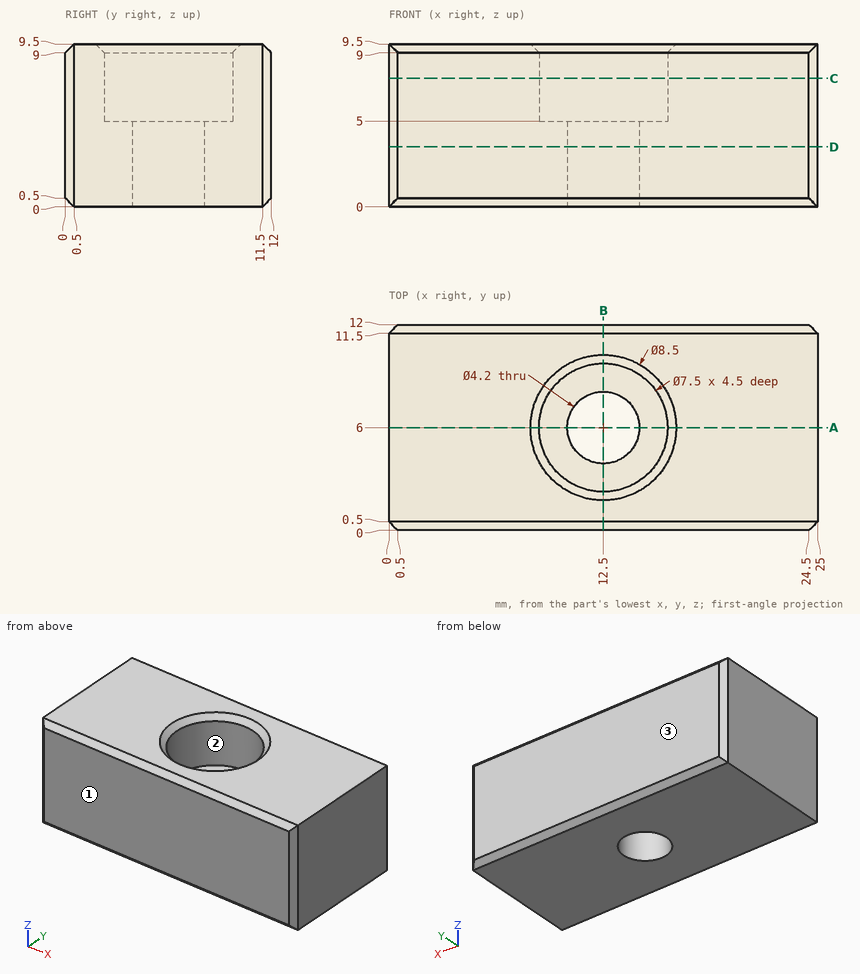
Here's the drawing with two shaded views (mm, measured from the low corner). I have some questions. Round coordinates to 2 decimals unless told otherwise and drop trailing zeros. Write each loop counter-clockwise with the first axis right and the second up, starting at its lowest first coordinate (ties: lowest second). Pieces come first, ordered by that corner, then holes.
(1) Suppose I cut it at C-C on z = 7.5. Write out the boundary of the cut face in (x, y).
Findings below:
outline: (0, 0.5) - (0.5, 0) - (24.5, 0) - (25, 0.5) - (25, 11.5) - (24.5, 12) - (0.5, 12) - (0, 11.5) - close; hole circle Ø7.5 at (12.5, 6)
(2) Suppose I cut it at D-D on z = 3.5. Write out the boundary of the cut face in (x, y), and give its area (3 significant figures).
Findings below:
outline: (0, 0.5) - (0.5, 0) - (24.5, 0) - (25, 0.5) - (25, 11.5) - (24.5, 12) - (0.5, 12) - (0, 11.5) - close; hole circle Ø4.2 at (12.5, 6)
area: 286 mm2
(3) Suppose I cut it at B-B on x = 12.5. Write out the boundary of the cut face in (y, z), and give its area (3 significant figures).
Findings below:
outline: (0, 0.5) - (0.5, 0) - (3.9, 0) - (3.9, 5) - (2.25, 5) - (2.25, 9) - (1.75, 9.5) - (0.5, 9.5) - (0, 9) - close; (8.1, 0) - (11.5, 0) - (12, 0.5) - (12, 9) - (11.5, 9.5) - (10.25, 9.5) - (9.75, 9) - (9.75, 5) - (8.1, 5) - close
area: 58.5 mm2
(4) For pin 1 (2 mm diameter, centred on x = 11, y = 5, fed in from +Z), with a flat end and sliding along its axis, tell me the tip position at first contact or that it passes through.
Findings below:
pin 1: stops at z = 5
(5) Suppose I cut it at A-A on y = 6. Write out the boundary of the cut face in (x, z).
Findings below:
outline: (0, 0) - (10.4, 0) - (10.4, 5) - (8.75, 5) - (8.75, 9) - (8.25, 9.5) - (0, 9.5) - close; (14.6, 0) - (25, 0) - (25, 9.5) - (16.75, 9.5) - (16.25, 9) - (16.25, 5) - (14.6, 5) - close
(6) Thinking about a two-plate mould opening in Y: for the marked faces 1, 2 and 3, which applies, +Y half, -Y half, draft (parallel to the pull), parting line (faces both ways), or undercut?
Findings below:
face 1: -Y half
face 2: undercut
face 3: +Y half
(7) If I drill on probe 1 along X at (y, z) = (6, 3.15); probe 2 along Y at (x, z) = (12.5, 7.55); probe 3 along X at (y, z) = (6, 6.15), over which ranges is the centre line in solid material (lowest first)?
Findings below:
probe 1: x = 0 to 10.4, 14.6 to 25
probe 2: y = 0 to 2.25, 9.75 to 12
probe 3: x = 0 to 8.75, 16.25 to 25
